from build123d import *

# Parameters (mm, degrees)
SKETCH1_W           = 55
SKETCH1_H           = 92.14389058
BOSS_EXTRUDE1_DEPTH = 2.5
BOSS_EXTRUDE2_DEPTH = 2.5
BOSS_EXTRUDE3_DEPTH = 2.5
FILLET1_R           = 1


with BuildPart() as part:
    # Sketch1 → Boss-Extrude1 (new body)
    with BuildSketch(Plane.XY):
        Rectangle(SKETCH1_W, SKETCH1_H)
    extrude(amount=BOSS_EXTRUDE1_DEPTH)

    # Sketch6 → Boss-Extrude2 (add, symmetric)
    with BuildSketch(Plane(origin=(0, 38.37194529, 0), x_dir=(1, 0, 0), z_dir=(0, 1, 0))):
        with BuildLine():
            Line((-4.053033857, -5), (-4.053033857, -2.5))
            Line((-4.053033857, -2.5), (4.053033857, -2.5))
            Line((4.053033857, -2.5), (4.053033857, -5))
            ThreePointArc((4.053033857, -5), (4.899562702, -7.805363596), (3.036123017, -10.066838454))
            Line((3.036123017, -10.066838454), (1.4, -10.066838454))
            Line((1.4, -10.066838454), (1.4, -5.066838454))
            ThreePointArc((1.4, -5.066838454), (1.111291087, -3.950394141), (0, -3.642444699))
            ThreePointArc((0, -3.642444699), (-1.111291087, -3.950394141), (-1.4, -5.066838454))
            Line((-1.4, -5.066838454), (-1.4, -10.066838454))
            Line((-1.4, -10.066838454), (-3.036123017, -10.066838454))
            ThreePointArc((-3.036123017, -10.066838454), (-4.899562702, -7.805363596), (-4.053033857, -5))
        make_face()
    extrude(amount=BOSS_EXTRUDE2_DEPTH, both=True)

    # Sketch7 → Boss-Extrude3 (add, symmetric)
    with BuildSketch(Plane(origin=(0, -40.22805471, 0), x_dir=(-1, 0, 0), z_dir=(0, -1, 0))):
        with BuildLine():
            Line((-4.053033857, -5), (-4.053033857, -2.5))
            Line((-4.053033857, -2.5), (4.053033857, -2.5))
            Line((4.053033857, -2.5), (4.053033857, -5))
            ThreePointArc((4.053033857, -5), (4.899562702, -7.805363596), (3.036123017, -10.066838454))
            Line((3.036123017, -10.066838454), (1.4, -10.066838454))
            Line((1.4, -10.066838454), (1.4, -5.066838454))
            ThreePointArc((1.4, -5.066838454), (1.111291087, -3.950394141), (0, -3.642444699))
            ThreePointArc((0, -3.642444699), (-1.111291087, -3.950394141), (-1.4, -5.066838454))
            Line((-1.4, -5.066838454), (-1.4, -10.066838454))
            Line((-1.4, -10.066838454), (-3.036123017, -10.066838454))
            ThreePointArc((-3.036123017, -10.066838454), (-4.899562702, -7.805363596), (-4.053033857, -5))
        make_face()
    extrude(amount=BOSS_EXTRUDE3_DEPTH, both=True)

    # Fillet1
    fillet1_edges = [part.edges().sort_by_distance(p)[0] for p in [
        (-27.5, 46.07194529, 1.25),
        (27.5, 46.07194529, 1.25),
        (27.5, -46.07194529, 1.25),
        (-27.5, -46.07194529, 1.25),
    ]]
    fillet(fillet1_edges, radius=FILLET1_R)


solid = part.part
Part model, mm, in its own coordinate system. A direction names the side the tool comes from. Coordinates: 2 decimals unless noted, no trailing zeros. Loops run counter-clockwise (first coordinate to the right, second up) from the corner with the lowest first, then second, coordinate; pieces in that order, holes last. Notation, with made-up numbers: (-28.5, 24.5) -> (12.5, 24.5) arc R22 cw to (12.5, 32.5) -> close; hole circle Ø3 at (89, 9). An arc over 180 degrees is marked (long way). Use a Markdown table: item, result. Add a question column.
Item 1: Band-saw the part on B-B on x = -11.5. Write the cut outline in (y, z).
Item 2: Band-saw the part on C-C on y = 37. Write the cut outline in (x, z).
Item 3: Probe probe 1 along Z at (x, y) = (-11.5, 18.5); probe 2 along X at (y, z) = (39.5, 9.75). List the from-to ranges inside material, lowest first.
Item 4: Flat gauge pins, fed straight in: P1, Ø1.2, axis at y = -40.5, z = 4, coming from the +X side; P2, Ø4, axis at y = -41, z = 7.5, coming from the -X side; P3, Ø2.5, axis at y = -41, z = 7.5, coming from the +X side. Where does each tip first touch, or does it go through?
Item 5: Band-saw the part on A-A on z = 9. Write the cut outline in (x, y).
Item 6: Band-saw the part on D-D on y = -2. Write the cut outline in (x, z).
Item 7: Which spindle directions (+Z, -Z, +X, -X, +Y, -Y) get a long thin tool onto all of the face, cutting with end or side? Do faces 1 (the flat face through (2, -42.728, 6)), 2 (the flat face through (-1.4, -40, 8)), 3 (the flat face through (4.053, -40, 4)), 4 (the flat face through (-4.053, -40, 4)). Say none if no direction does.
Geometry says:
| question | item | result |
|---|---|---|
| 1 | outline | (-46.07, 0) -> (46.07, 0) -> (46.07, 2.5) -> (-46.07, 2.5) -> close |
| 2 | outline | (-27.5, 0) -> (27.5, 0) -> (27.5, 2.5) -> (4.05, 2.5) -> (4.05, 5) arc R3.11 ccw to (3.04, 10.07) -> (1.4, 10.07) -> (1.4, 5.07) arc R1.15 cw to (0, 3.64) arc R1.15 cw to (-1.4, 5.07) -> (-1.4, 10.07) -> (-3.04, 10.07) arc R3.11 ccw to (-4.05, 5) -> (-4.05, 2.5) -> (-27.5, 2.5) -> close |
| 3 | probe 1 | 0 to 2.5 |
| 3 | probe 2 | -3.62 to -1.4, 1.4 to 3.62 |
| 4 | P1 | x = 4.05 |
| 4 | P2 | x = -4.96 |
| 4 | P3 | x = 4.96 |
| 5 | outline | (-4.38, -42.73) -> (-1.4, -42.73) -> (-1.4, -37.73) -> (-4.38, -37.73) -> close; (-4.38, 35.87) -> (-1.4, 35.87) -> (-1.4, 40.87) -> (-4.38, 40.87) -> close; (1.4, -42.73) -> (4.38, -42.73) -> (4.38, -37.73) -> (1.4, -37.73) -> close; (1.4, 35.87) -> (4.38, 35.87) -> (4.38, 40.87) -> (1.4, 40.87) -> close |
| 6 | outline | (-27.5, 0) -> (27.5, 0) -> (27.5, 2.5) -> (-27.5, 2.5) -> close |
| 7 | face 1 | +Z, +X, -X, -Y |
| 7 | face 2 | +Z, +Y, -Y |
| 7 | face 3 | +X, +Y, -Y |
| 7 | face 4 | -X, +Y, -Y |
